The model under review builds one solid part; all positions refer to its coordinate system, in mm. Coordinates: 2 decimals unless noted, no trailing zeros. Order: outer loops, then holes, each group sorted by start corner. A loop starts at its lowest first (then second) coordinate and runs counter-clockwise, first axis right, second up. Notation, with made-up numbers: (5.25, 23.25) - (61.25, 23.25) arc R28 cw to (61.25, 47.25) - close; hole circle Ø5 at (-18.75, 75). An arc over 180 degrees is marked (long way). Answer in a Markdown table with one row per item.
```python
from build123d import *

# Parameters (mm, degrees)
SKETCH1_R                      = 27
BOSS_EXTRUDE1_DEPTH            = 8
M5_CLEARANCE_HOLE1_D           = 5.5
M5_CLEARANCE_HOLE1_CSINK_D     = 5.55
M5_CLEARANCE_HOLE1_CSINK_ANGLE = 90


with BuildPart() as part:
    # Sketch1 → Boss-Extrude1 (new body)
    with BuildSketch(Plane(origin=(0, 0, 0), x_dir=(1, 0, 0), z_dir=(0, 1, 0))):
        with Locations(Location((0, 0, 0), (0, 0, 270))):
            Circle(SKETCH1_R)
    extrude(amount=BOSS_EXTRUDE1_DEPTH)

    # M5 Clearance Hole1 (through all)
    with Locations(Plane(origin=(0, 8, 0), x_dir=(1, 0, 0), z_dir=(0, 1, 0))):
        with Locations((-6.92820323, 4), (6.92820323, 4), (0, -8)):
            CounterSinkHole(M5_CLEARANCE_HOLE1_D / 2, M5_CLEARANCE_HOLE1_CSINK_D / 2, counter_sink_angle=M5_CLEARANCE_HOLE1_CSINK_ANGLE)


solid = part.part
```
Item 1: We need section A-A, the plane x = 0. Write out the cut boundary in (y, z) (3 decimals), then the cut area to 3 significant figures.
Check values:
| item | result |
|---|---|
| outline | (0, -27) - (8, -27) - (8, 5.225) - (7.975, 5.25) - (0, 5.25) - close; (0, 10.75) - (7.975, 10.75) - (8, 10.775) - (8, 27) - (0, 27) - close |
| area | 388 mm^2 |
Item 2: We need section B-B, the plane z = -4. Write out the cut boundary in (x, y) (3 decimals), then the cut area to 3 significant figures.
Check values:
| item | result |
|---|---|
| outline | (-26.702, 0) - (-9.678, 0) - (-9.678, 7.975) - (-9.703, 8) - (-26.702, 8) - close; (-4.178, 0) - (4.178, 0) - (4.178, 7.975) - (4.153, 8) - (-4.153, 8) - (-4.178, 7.975) - close; (9.678, 0) - (26.702, 0) - (26.702, 8) - (9.703, 8) - (9.678, 7.975) - close |
| area | 339 mm^2 |
Item 3: We need section C-C, the plane y = 0.75. Write out the cut boundary in (x, z), then the cut area to 3 significant figures.
Check values:
| item | result |
|---|---|
| outline | circle Ø54 at (0, 0); hole circle Ø5.5 at (-6.93, -4); hole circle Ø5.5 at (0, 8); hole circle Ø5.5 at (6.93, -4) |
| area | 2,220 mm^2 |
Item 4: Clearance check with flat-ended pins moving along their axes: pin 1 Ø6.5 at (x, z) = (0, 8) entering from +Y; pin 2 Ø1.5 at (y, z) = (5.5, 10.5) entering from -X; pin 3 Ø1.5 at (y, z) = (5.5, 6) entering from +X; pin 4 Ø2 at (x, y) = (-19.5, 5.5) entering from -Z. State where each tip first meets the part, or that it passes through.
Check values:
| item | result |
|---|---|
| pin 1 | y = 8 |
| pin 2 | x = -25.18 |
| pin 3 | x = 26.48 |
| pin 4 | z = -19.67 |
Item 5: To check wall thickness, follow line 1 (Z direction, x = 1.5, y = 3.5); line 2 (X direction, y = 1, z = -2.5); line 3 (X direction, y = 4, z = 0.5). State the ranges of each line that lie inside material, in increasing order. Write a range as from..to.
Check values:
| item | result |
|---|---|
| line 1 | -26.96..5.7, 10.3..26.96 |
| line 2 | -26.88..-9.23, -4.62..4.62, 9.23..26.88 |
| line 3 | -27..27 |
Item 6: Mouldability with a two-part tool opening along X and no side actions: class faces 1 (the face through (-26.36, 3.94, -5.85)), 2 (the face through (7.524, 3.932, -1.315)), 3 (the face through (0, 8, 0)) as +X half, -X half, draft (parallel to the pull), parting line (faces both ways), or undercut.
Check values:
| item | result |
|---|---|
| face 1 | parting line |
| face 2 | undercut |
| face 3 | draft |
Item 7: We need section D-D, the plane z = 8. Write out the cut boundary in (x, y) (3 decimals), then the cut area to 3 significant figures.
Check values:
| item | result |
|---|---|
| outline | (-25.788, 0) - (-2.75, 0) - (-2.75, 7.975) - (-2.775, 8) - (-25.788, 8) - close; (2.75, 0) - (25.788, 0) - (25.788, 8) - (2.775, 8) - (2.75, 7.975) - close |
| area | 369 mm^2 |
